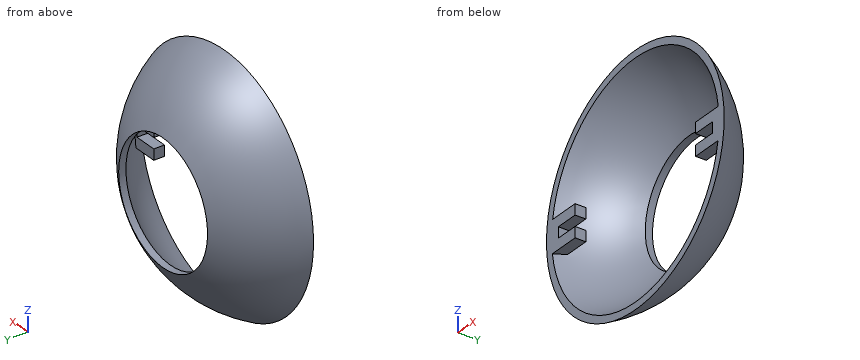
```python
from build123d import *

# Parameters (mm, degrees)
SALIENTE_EXTRUIR1_DEPTH = 5


with BuildPart() as part:
    # Croquis2 → Revolución2 (revolve)
    with BuildSketch(Plane.XY):
        with BuildLine():
            Line((57, 27.986603938), (53.637673328, 27.986603938))
            ThreePointArc((53.637673328, 27.986603938), (42.984719481, 42.574216272), (28.5, 53.366656257))
            Line((28.5, 53.366656257), (28.5, 56.745043836))
            ThreePointArc((28.5, 56.745043836), (45.103486188, 44.698160294), (57, 27.986603938))
        make_face()
    revolve(axis=Axis((0, 10.058437275, 0), (0, 1, 0)))

    # Croquis3 → Saliente-Extruir1 (add)
    with BuildSketch(Plane.XZ.offset(-27.986603938)):
        with BuildLine():
            Line((38.630056924, 1.848931625), (49.379751122, 1.848931625))
            Line((49.379751122, 1.848931625), (49.379751122, -3.151068375))
            Line((49.379751122, -3.151068375), (38.630056924, -3.151068375))
            Line((38.630056924, -3.151068375), (38.630056924, -8.151068375))
            Line((38.630056924, -8.151068375), (53.014715734, -8.151068375))
            ThreePointArc((53.014715734, -8.151068375), (53.633642946, -0.657528958), (53.198610279, 6.848931625))
            Line((53.198610279, 6.848931625), (38.630056924, 6.848931625))
            Line((38.630056924, 6.848931625), (38.630056924, 1.848931625))
        make_face()
        with BuildLine():
            Line((-38.630056924, 8.151068375), (-53.014715734, 8.151068375))
            ThreePointArc((-53.014715734, 8.151068375), (-53.633642946, 0.657528958), (-53.198610279, -6.848931625))
            Line((-53.198610279, -6.848931625), (-38.630056924, -6.848931625))
            Line((-38.630056924, -6.848931625), (-38.630056924, -1.848931625))
            Line((-38.630056924, -1.848931625), (-49.379751122, -1.848931625))
            Line((-49.379751122, -1.848931625), (-49.379751122, 3.151068375))
            Line((-49.379751122, 3.151068375), (-38.630056924, 3.151068375))
            Line((-38.630056924, 3.151068375), (-38.630056924, 8.151068375))
        make_face()
    extrude(amount=-SALIENTE_EXTRUIR1_DEPTH)


solid = part.part
```
Input: part model. Units: mm. Frame: model coordinates. Coordinates: 2 decimals unless noted, no trailing zeros. Loops run counter-clockwise (first coordinate to the right, second up) from the corner with the lowest first, then second, coordinate; pieces in that order, holes last. Notation, with made-up numbers: M 85.5,66 L 141.5,66 A20 cw 141.5,105 Z; hole C 21,25.5 d10. An arc over 180 degrees is marked long. Answer in a Markdown table with one row per item.
1. Section B-B, the plane x = 0. Output: boundary loops of the cut face in (y, z).
Response:
| item | result |
|---|---|
| outline | M 27.99,-57 A63.5 ccw 56.75,-28.5 L 53.37,-28.5 A60.5 cw 27.99,-53.64 Z; M 27.99,53.64 A60.5 cw 53.37,28.5 L 56.75,28.5 A63.5 ccw 27.99,57 Z |
2. Material intervals for line 1 (Z direction, x = 0, y = 54.85); line 2 (X direction, y = 43.25, z = -20.5); line 3 (Z direction, x = 36.5, y = 40.75), sorted ascending.
Response:
| item | result |
|---|---|
| line 1 | z = -32 to -28.5, 28.5 to 32 |
| line 2 | x = -41.73 to -37.01, 37.01 to 41.73 |
| line 3 | z = -32.24 to -25.83, 25.83 to 32.24 |
3. Section C-C, the plane x = -46. Output: boundary loops of the cut face in (y, z) (3 decimals).
Response:
| item | result |
|---|---|
| outline | M 27.987,-33.66 A43.775 ccw 27.987,33.66 L 27.987,27.586 A39.297 cw 27.987,-27.586 Z; M 27.987,-6.849 L 32.987,-6.849 L 32.987,-1.849 L 27.987,-1.849 Z; M 27.987,3.151 L 32.987,3.151 L 32.987,8.151 L 27.987,8.151 Z |
4. Section A-A, the plane z = 0. Output: boundary loops of the cut face in (x, y), then the cut area to 3 significant figures.
Response:
| item | result |
|---|---|
| outline | M -57,27.99 L -49.38,27.99 L -49.38,32.99 L -50.72,32.99 A60.5 cw -28.5,53.37 L -28.5,56.75 A63.5 ccw Z; M 28.5,53.37 A60.5 cw 50.72,32.99 L 49.38,32.99 L 49.38,27.99 L 57,27.99 A63.5 ccw 28.5,56.75 Z |
| area | 261 mm2 |
5. First-contact query: pin 1 (4 mm diameter, centred on y = 33, z = 1, fed in from +X); pin 2 (5.5 mm diameter, centred on x = 46, y = 30.5, fed in from +Z) (3 decimals); pin 3 (1.5 mm diameter, centred on x = 11.5, z = -40, fed in from +Y). Flat tips, straight axial feed; report the tip coordinate or a pass-through.
Response:
| item | result |
|---|---|
| pin 1 | stops at x = 55.41 |
| pin 2 | stops at z = 35.805 |
| pin 3 | stops at y = 48.6 |
6. Section D-D, the plane z = -25.5. Output: boundary loops of the cut face in (x, y).
Response:
| item | result |
|---|---|
| outline | M -50.98,27.99 L -47.19,27.99 A54.86 cw -12.73,53.37 L -12.73,56.75 A58.15 ccw Z; M 12.73,53.37 A54.86 cw 47.19,27.99 L 50.98,27.99 A58.15 ccw 12.73,56.75 Z |
